Source: CAD feature listing. Evaluate the final solid. Frame: model axes, mm. Face numbers are marked on the shaded views. A direction names the side the tool comes from. Give positions to 0.01 mm unless a question says otherwise; leave off trailing zeros. Order: outer loops, then holes, each group sorted by start corner. A loop starts at its lowest first (then second) coordinate and runs counter-clockwise, first axis right, second up. Notation, with made-up numbers: (-7.5, 37) - (10.5, 37) arc R12 ccw to (10.5, 44) - close; hole circle Ø10 at (-3.5, 18.5). An arc over 180 degrees is marked (long way). One line per item, written item: value. Start each with the question number.
from build123d import *

# Parameters (mm, degrees)
SKETCH1_W           = 12.7
SKETCH1_H           = 2.54
BOSS_EXTRUDE1_DEPTH = 38.1
SKETCH3_W           = 38.1
SKETCH3_H           = 2.54
CUT_EXTRUDE1_DEPTH  = 2.54
SKETCH4_W           = 38.1
SKETCH4_H           = 2.54
CUT_EXTRUDE2_DEPTH  = 2.54
SKETCH5_W           = 2.54
SKETCH5_H           = 38.1
BOSS_EXTRUDE3_DEPTH = 2.54


with BuildPart() as part:
    # Sketch1 → Boss-Extrude1 (new body)
    with BuildSketch(Plane.XY):
        Rectangle(SKETCH1_W, SKETCH1_H)
    extrude(amount=BOSS_EXTRUDE1_DEPTH)

    # Sketch3 → Cut-Extrude1 (cut)
    with BuildSketch(Plane(origin=(6.35, 0, 0), x_dir=(0, 0, -1), z_dir=(1, 0, 0))):
        with Locations((-19.05, 0)):
            Rectangle(SKETCH3_W, SKETCH3_H)
    extrude(amount=-CUT_EXTRUDE1_DEPTH, mode=Mode.SUBTRACT)

    # Sketch4 → Cut-Extrude2 (cut)
    with BuildSketch(Plane.ZY.offset(6.35)):
        with Locations((19.05, 0)):
            Rectangle(SKETCH4_W, SKETCH4_H)
    extrude(amount=-CUT_EXTRUDE2_DEPTH, mode=Mode.SUBTRACT)

    # Sketch5 → Boss-Extrude3 (add)
    with BuildSketch(Plane(origin=(0, 1.27, 0), x_dir=(1, 0, 0), z_dir=(0, 1, 0))):
        with Locations((0, -19.05)):
            Rectangle(SKETCH5_W, SKETCH5_H)
    extrude(amount=BOSS_EXTRUDE3_DEPTH)


solid = part.part
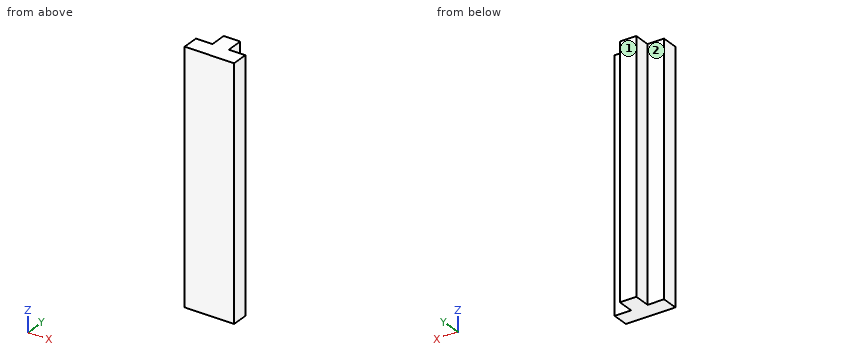
1. Section B-B on x = -2.75. Return the cut outline in (y, z).
2. Set-up query: the marked faces 1 and 2. Return all of +Z, -Z, +X, -X, +Y, -Y with unobstructed straight access to the full face (end or side cutting, diameter ignored); none if empty.
3. Contact query for flat-ended pins moving along their axis: pin 1 Ø0.8 at (x, z) = (-2, 12) entering from +Y; pin 2 Ø3 at (x, z) = (2.5, 17) entering from +Y; pin 3 Ø0.8 at (y, z) = (2.5, 28) entering from +X; pin 4 Ø1.5 at (x, y) = (3, 3) entering from +Z. Output: stop coordinate, or through.
4. Ray query, L1, parallel to X at y = 2.75, z = 26.5. Return the intervals inside material, ascending.
5. Section A-A on z = 20. Return the cut outline in (x, y), then the cut area to 3 significant figures.
Data:
1. outline: (-1.27, 0) - (1.27, 0) - (1.27, 38.1) - (-1.27, 38.1) - close
2. face 1: +Z, -Z, +X, -X, +Y
2. face 2: +Z, -Z, -X, +Y
3. pin 1: stops at y = 1.27
3. pin 2: stops at y = 3.81
3. pin 3: stops at x = 1.27
3. pin 4: passes through
4. L1: x = -1.27 to 1.27
5. outline: (-3.81, -1.27) - (3.81, -1.27) - (3.81, 1.27) - (1.27, 1.27) - (1.27, 3.81) - (-1.27, 3.81) - (-1.27, 1.27) - (-3.81, 1.27) - close
5. area: 25.8 mm2
